For this review, take the finished solid that the model builds, in its own axes (mm). Give positions to 0.01 mm unless a question says otherwise; leave off trailing zeros. Write each loop counter-clockwise with the first axis right and the second up, starting at its lowest first coordinate (ties: lowest second). Pieces come first, ordered by that corner, then holes. Notation, with made-up numbers: M 80,87.25 L 100,87.25 A12 ccw 100,104.25 Z; hole C -14,64 d4. An arc over 180 degrees is marked long. Use one line per item in the form item = value. Start each with the question number.
Q1. Consider section C-C on z = 0. Write out the cut boundary in (x, y).
Q2. Consider section D-D on y = -3.25. Give the number of separate pieces and of enclosed holes in the cut face, and give its area (3 significant figures).
Q3. Consider section B-B on x = 60. Write out the cut boundary in (y, z), and give its area (3 significant figures).
Q4. Clearance check with a flat-ended pin moving along its axis: pin 1 Ø1.5 at (x, z) = (49, -33) entering from +Y. State where the tip first meets the part, or that it passes through.
Q5. For probe 1 along X at (y, z) = (-5, 0); probe 2 along X at (y, z) = (-5.5, -31); probe 3 along Z at (x, y) = (-0.5, -3.5), list the stretches that pass through material, from the lowest coordinate up. Write a range as [from, to].
Q6. Consider section A-A on z = -37.5. Write out the cut boundary in (x, y), and give its area (3 significant figures).
Q7. Mouldability with a two-part tool opening along Z and no side actions: class faces 1 (the flat face through (32, -3, 42.5)), 2 (the cylindrical face through (-39.55, -3.13, -0.46)), 3 (the cylindrical face through (-42.49, -3.13, -0.93)), 4 (the cylindrical face through (58.722, -3.131, 30.834)) as released by +Z, released by -Z, zero draft, split by the parting line, or undercut.
```python
from build123d import *

# Parameters (mm, degrees)
SKETCH1_R           = 2.1
SKETCH1_R_2         = 10
BOSS_EXTRUDE1_DEPTH = 6.35


with BuildPart() as part:
    # Sketch1 → Boss-Extrude1 (new body)
    with BuildSketch(Plane(origin=(0, 0, 0), x_dir=(1, 0, 0), z_dir=(0, 1, 0))):
        with BuildLine():
            Line((65, 42.5), (0, 42.5))
            ThreePointArc((0, 42.5), (-42.5, 0), (0, -42.5))
            Line((0, -42.5), (65, -42.5))
            Line((65, -42.5), (65, 42.5))
        make_face()
        with Locations(Location((40, -32.5, 0), (0, 0, 270))):
            Circle(SKETCH1_R, mode=Mode.SUBTRACT)
        with Locations(Location((60, -32.5, 0), (0, 0, 270))):
            Circle(SKETCH1_R, mode=Mode.SUBTRACT)
        with Locations(Location((40, 32.5, 0), (0, 0, 270))):
            Circle(SKETCH1_R, mode=Mode.SUBTRACT)
        with Locations(Location((60, 32.5, 0), (0, 0, 270))):
            Circle(SKETCH1_R, mode=Mode.SUBTRACT)
        with Locations(Location((37.5, 0, 0), (0, 0, 270))):
            Circle(SKETCH1_R, mode=Mode.SUBTRACT)
        with Locations(Location((17.67766953, 17.67766953, 0), (0, 0, 270))):
            Circle(SKETCH1_R, mode=Mode.SUBTRACT)
        with Locations(Location((0, -37.5, 0), (0, 0, 270))):
            Circle(SKETCH1_R, mode=Mode.SUBTRACT)
        with Locations(Location((-17.67766953, -17.67766953, 0), (0, 0, 270))):
            Circle(SKETCH1_R, mode=Mode.SUBTRACT)
        with Locations(Location((17.67766953, -17.67766953, 0), (0, 0, 270))):
            Circle(SKETCH1_R, mode=Mode.SUBTRACT)
        with Locations(Location((-37.5, 0, 0), (0, 0, 270))):
            Circle(SKETCH1_R, mode=Mode.SUBTRACT)
        with Locations(Location((-17.67766953, 17.67766953, 0), (0, 0, 270))):
            Circle(SKETCH1_R, mode=Mode.SUBTRACT)
        with Locations(Location((0, 0, 0), (0, 0, 270))):
            Circle(SKETCH1_R_2, mode=Mode.SUBTRACT)
        with Locations(Location((0, 37.5, 0), (0, 0, 270))):
            Circle(SKETCH1_R, mode=Mode.SUBTRACT)
    extrude(amount=-BOSS_EXTRUDE1_DEPTH)


solid = part.part
```
Working result:
q1.outline = M -42.5,-6.35 L -39.6,-6.35 L -39.6,0 L -42.5,0 Z; M -35.4,-6.35 L -10,-6.35 L -10,0 L -35.4,0 Z; M 10,-6.35 L 35.4,-6.35 L 35.4,0 L 10,0 Z; M 39.6,-6.35 L 65,-6.35 L 65,0 L 39.6,0 Z
q2.separate_pieces = 1
q2.enclosed_holes = 13
q2.area = 7,880 mm²
q3.outline = M -6.35,-42.5 L 0,-42.5 L 0,-34.6 L -6.35,-34.6 Z; M -6.35,-30.4 L 0,-30.4 L 0,30.4 L -6.35,30.4 Z; M -6.35,34.6 L 0,34.6 L 0,42.5 L -6.35,42.5 Z
q3.area = 486 mm²
q4.pin_1 = 0
q5.probe_1 = [-42.5, -39.6], [-35.4, -10], [10, 35.4], [39.6, 65]
q5.probe_2 = [-29.07, 38.53], [41.47, 58.53], [61.47, 65]
q5.probe_3 = [-42.5, -39.54], [-35.46, -9.99], [9.99, 35.46], [39.54, 42.5]
q6.outline = M -20,-6.35 L -2.1,-6.35 L -2.1,0 L -20,0 Z; M 2.1,-6.35 L 65,-6.35 L 65,0 L 2.1,0 Z
q6.area = 513 mm²
q7.face_1 = released by +Z
q7.face_2 = undercut
q7.face_3 = split by the parting line
q7.face_4 = undercut
